Source: CAD feature listing. Evaluate the final solid. Frame: model axes, mm. Face numbers are marked on the shaded views. A direction names the side the tool comes from. Give positions to 0.01 mm unless a question says otherwise; leave off trailing zeros. Order: outer loops, then holes, each group sorted by start corner. A loop starts at its lowest first (then second) coordinate and runs counter-clockwise, first axis right, second up. Notation, with made-up numbers: (49, 89) -> (81, 89) arc R18 ccw to (81, 108) -> close; hole circle Ø7 at (-17, 87). An arc over 180 degrees is marked (long way). Answer in a Markdown table with one row per item.
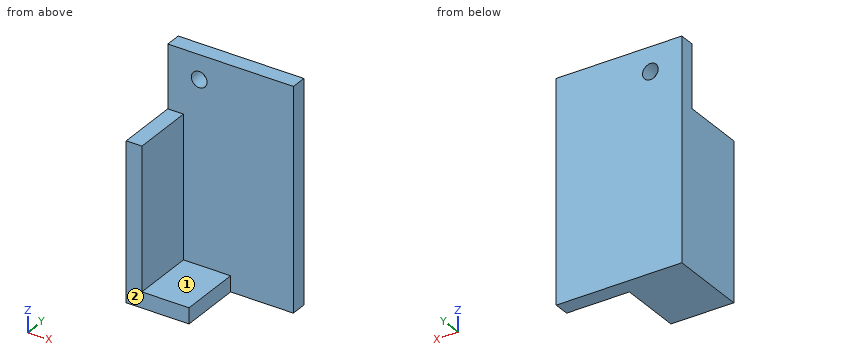
```python
from build123d import *

# Parameters (mm, degrees)
F0_W     = 50.8
F0_H     = 88.9
F1_DEPTH = 31.75
F2_W     = 25.4
F2_H     = 82.55
F3_DEPTH = 44.45
F4_W     = 25.4
F4_H     = 25.4
F5_DEPTH = 25.4
F6_W     = 25.4
F6_H     = 6.35
F7_DEPTH = 25.4
F8_R     = 3.175
F9_DEPTH = 25.4


with BuildPart() as f1:
    # F0 (on Front) → F1 (new body)
    with BuildSketch(Plane.XZ):
        Rectangle(F0_W, F0_H)
    extrude(amount=F1_DEPTH)

    # F2 (on face) → F3 (cut)
    with BuildSketch(Plane.YZ.offset(25.4)):
        with Locations((-19.05, 3.175)):
            Rectangle(F2_W, F2_H)
    extrude(amount=-F3_DEPTH, mode=Mode.SUBTRACT)

    # F4 (on face) → F5 (cut)
    with BuildSketch(Plane(origin=(-25.4, 0, 0), x_dir=(0, -1, 0), z_dir=(-1, 0, 0))):
        with Locations((19.05, 31.75)):
            Rectangle(F4_W, F4_H)
    extrude(amount=-F5_DEPTH, mode=Mode.SUBTRACT)

    # F6 (on face) → F7 (cut)
    with BuildSketch(Plane.XZ.offset(31.75)):
        with Locations((12.7, -41.275)):
            Rectangle(F6_W, F6_H)
    extrude(amount=-F7_DEPTH, mode=Mode.SUBTRACT)

    # F8 (on face) → F9 (cut)
    with BuildSketch(Plane(origin=(0, 0, 0), x_dir=(-1, 0, 0), z_dir=(0, 1, 0))):
        with Locations((12.7, 34.658268)):
            Circle(F8_R)
    extrude(amount=-F9_DEPTH, mode=Mode.SUBTRACT)


solid = f1.part
```
(1) Section query C-C (z = 0.5). Return the cut outline in (x, y).
A:
| item | result |
|---|---|
| outline | (-25.4, -31.75) -> (-19.05, -31.75) -> (-19.05, -6.35) -> (25.4, -6.35) -> (25.4, 0) -> (-25.4, 0) -> close |
(2) Ray query, probe 1 along Z at (x, y) = (-12.7, -4.5); probe 2 along X at (y, z) = (-22.5, -3); probe 3 along Y at (x, z) = (8.5, -6.5). Return the intervals inside material, ascending.
A:
| item | result |
|---|---|
| probe 1 | z = -44.45 to 31.48, 37.83 to 44.45 |
| probe 2 | x = -25.4 to -19.05 |
| probe 3 | y = -6.35 to 0 |
(3) First-contact query: pin 1 Ø8 at (x, y) = (3, -14.5) entering from +Z; pin 2 Ø3 at (y, z) = (-15, -40) entering from +X; pin 3 Ø10 at (x, z) = (9.5, -34.5) entering from -Y. Flat tips, straight axial feed; report the tip coordinate or a pass-through.
A:
| item | result |
|---|---|
| pin 1 | stops at z = -38.1 |
| pin 2 | stops at x = 0 |
| pin 3 | stops at y = -6.35 |
(4) Access query for the marked faces 1 and 2. Directions: +Z, -Z, +X, -X, +Y, -Y. A direction counts if a zero-diameter tool reaches every point of the face in a straight line with its end or side. Return the directions, or none.
A:
| item | result |
|---|---|
| face 1 | +Z, +X, -Y |
| face 2 | +Z, -Z, +X, -X, -Y |
(5) Section query D-D (x = 11.5). Return the cut outline in (y, z), plus the area to 3 significant figures.
A:
| item | result |
|---|---|
| outline | (-6.35, -44.45) -> (0, -44.45) -> (0, 44.45) -> (-6.35, 44.45) -> close |
| area | 565 mm^2 |
(6) Section query A-A (x = -12.7). Return the cut outline in (y, z).
A:
| item | result |
|---|---|
| outline | (-31.75, -44.45) -> (0, -44.45) -> (0, 31.48) -> (-6.35, 31.48) -> (-6.35, -38.1) -> (-31.75, -38.1) -> close; (-6.35, 37.83) -> (0, 37.83) -> (0, 44.45) -> (-6.35, 44.45) -> close |
(7) Section query B-B (y = -9). Return the cut outline in (x, z), plus the area to 3 significant figures.
A:
| item | result |
|---|---|
| outline | (-25.4, -44.45) -> (0, -44.45) -> (0, -38.1) -> (-19.05, -38.1) -> (-19.05, 19.05) -> (-25.4, 19.05) -> close |
| area | 524 mm^2 |
